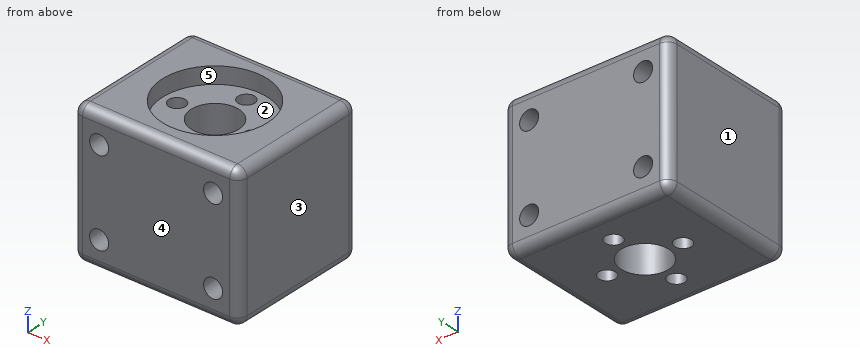
from build123d import *

# Parameters (mm, degrees)
CROQUIS1_W                 = 35
CROQUIS1_H                 = 30
CROQUIS1_R                 = 5
CROQUIS1_R_2               = 1.75
SALIENTE_EXTRUIR1_DEPTH    = 30
CROQUIS2_R                 = 11
CORTAR_EXTRUIR1_DEPTH      = 3.5
REDONDEO2_R                = 2
CORTAR_EXTRUIR2_DEPTH      = 10
CORTAR_EXTRUIR2_DEPTH_BACK = 31.5
CROQUIS3_R                 = 2


with BuildPart() as part:
    # Croquis1 → Saliente-Extruir1 (new body)
    with BuildSketch(Plane.XY):
        Rectangle(CROQUIS1_W, CROQUIS1_H)
        Circle(CROQUIS1_R, mode=Mode.SUBTRACT)
        with Locations((0, 8)):
            Circle(CROQUIS1_R_2, mode=Mode.SUBTRACT)
        with Locations((8, 0)):
            Circle(CROQUIS1_R_2, mode=Mode.SUBTRACT)
        with Locations((0, -8)):
            Circle(CROQUIS1_R_2, mode=Mode.SUBTRACT)
        with Locations((-8, 0)):
            Circle(CROQUIS1_R_2, mode=Mode.SUBTRACT)
    extrude(amount=SALIENTE_EXTRUIR1_DEPTH)

    # Croquis2 → Cortar-Extruir1 (cut)
    with BuildSketch(Plane.XY.offset(30)):
        Circle(CROQUIS2_R)
    extrude(amount=-CORTAR_EXTRUIR1_DEPTH, mode=Mode.SUBTRACT)

    # Redondeo2
    redondeo2_edges = [part.edges().sort_by_distance(p)[0] for p in [
        (-17.5, 0, 30),
        (0, -15, 30),
        (17.5, 0, 30),
        (0, -15, 0),
        (-17.5, 0, 0),
        (0, 15, 0),
        (17.5, 0, 0),
        (17.5, -15, 15),
        (-17.5, -15, 15),
        (-17.5, 15, 15),
        (17.5, 15, 15),
        (0, 15, 30),
    ]]
    fillet(redondeo2_edges, radius=REDONDEO2_R)

    # Croquis3 → Cortar-Extruir2 (cut, two sides: drawn at the far end of the back side and taken through both)
    with BuildSketch(Plane(origin=(0, 15, 0), x_dir=(1, 0, 0), z_dir=(0, 1, 0)).offset(-CORTAR_EXTRUIR2_DEPTH_BACK)):
        with Locations(Location((-12, -24, 0), (0, 0, 90))):
            Circle(CROQUIS3_R)
        with Locations(Location((12, -24, 0), (0, 0, 90))):
            Circle(CROQUIS3_R)
        with Locations(Location((-12, -6, 0), (0, 0, 90))):
            Circle(CROQUIS3_R)
        with Locations(Location((12, -6, 0), (0, 0, 90))):
            Circle(CROQUIS3_R)
    extrude(amount=CORTAR_EXTRUIR2_DEPTH + CORTAR_EXTRUIR2_DEPTH_BACK, mode=Mode.SUBTRACT)


solid = part.part
Read the model definition and answer for the solid it produces. Units are mm, in the model's axes. Face numbers are marked on the shaded views. A direction names the side the tool comes from. Coordinates: 2 decimals unless noted, no trailing zeros. Order: outer loops, then holes, each group sorted by start corner. A loop starts at its lowest first (then second) coordinate and runs counter-clockwise, first axis right, second up. Notation, with made-up numbers: M 25,18 L 61,18 A5 cw 61,27 Z; hole C 14.5,71 d6. An arc over 180 degrees is marked long. Put each result on its own line as item: value. Start each with the question number.
Item 1: The mould has two halves that part along X. Classify the marked faces 1, 2 and 3: +X half, -X half, draft (parallel to the pull), parting line (faces both ways), or undercut.
Item 2: For the marked faces 4 and 5, determine the directions among +Z, -Z, +X, -X, +Y, -Y from which every point of the face is accessible in a straight line to the end or side of a thin tool.
Item 3: Given pin 1 Ø13 at (x, y) = (0, 0) entering from +Z, flat-ended and moving along its own axis, determine where the tip first touches the part or whether it passes through.
Item 4: Section C-C, the plane z = 27 is taken. Determine the outline of the cut face in (x, y).
Item 5: Section B-B, the plane x = -12 is taken. Determine the outline of the cut face in (y, z), plus the area to 3 significant figures.
Item 6: Consider probe 1 along X at (y, z) = (0, 20.25); probe 2 along Y at (x, z) = (0, 19); probe 3 along X at (y, z) = (-1, 19.5). Determine where each line is inside the solid, lowest interval first. Write a range as [from, to].
Item 7: Section A-A, the plane y = -3.5 is taken. Determine the outline of the cut face in (x, z), plus the area to 3 significant figures.
Item 8: Section D-D, the plane y = 0 is taken. Determine the outline of the cut face in (x, z), plus the area to 3 significant figures.
Computed:
1. face 1: -X half
1. face 2: undercut
1. face 3: +X half
2. face 4: +Z, -Z, +X, -X, -Y
2. face 5: +Z
3. pin 1: stops at z = 26.5
4. outline: M -17.5,-13 A2 ccw -15.5,-15 L 15.5,-15 A2 ccw 17.5,-13 L 17.5,13 A2 ccw 15.5,15 L -15.5,15 A2 ccw -17.5,13 Z; hole C 0,0 d22
5. outline: M -15,2 A2 ccw -13,0 L 13,0 A2 ccw 15,2 L 15,4 L -15,4 Z; M -15,8 L 15,8 L 15,22 L -15,22 Z; M -15,26 L 15,26 L 15,28 A2 ccw 13,30 L -13,30 A2 ccw -15,28 Z
5. area: 657 mm2
6. probe 1: x = [-17.5, -9.75], [-6.25, -5], [5, 6.25], [9.75, 17.5]
6. probe 2: y = [-15, -9.75], [-6.25, -5], [5, 6.25], [9.75, 15]
6. probe 3: x = [-17.5, -9.44], [-6.56, -4.9], [4.9, 6.56], [9.44, 17.5]
7. outline: M -17.5,2 A2 ccw -15.5,0 L -3.57,0 L -3.57,26.5 L -10.43,26.5 L -10.43,30 L -15.5,30 A2 ccw -17.5,28 Z; M 3.57,0 L 15.5,0 A2 ccw 17.5,2 L 17.5,28 A2 ccw 15.5,30 L 10.43,30 L 10.43,26.5 L 3.57,26.5 Z; hole C -12,6 d4; hole C -12,24 d4; hole C 12,6 d4; hole C 12,24 d4
7. area: 734 mm2
8. outline: M -17.5,2 A2 ccw -15.5,0 L -9.75,0 L -9.75,26.5 L -11,26.5 L -11,30 L -15.5,30 A2 ccw -17.5,28 Z; M -6.25,0 L -5,0 L -5,26.5 L -6.25,26.5 Z; M 5,0 L 6.25,0 L 6.25,26.5 L 5,26.5 Z; M 9.75,0 L 15.5,0 A2 ccw 17.5,2 L 17.5,28 A2 ccw 15.5,30 L 11,30 L 11,26.5 L 9.75,26.5 Z; hole C -12,6 d4; hole C -12,24 d4; hole C 12,6 d4; hole C 12,24 d4
8. area: 469 mm2
